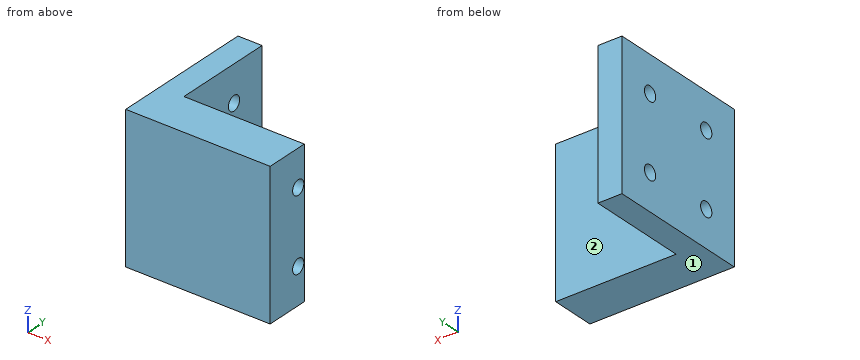
```python
from build123d import *

# Parameters (mm, degrees)
SKETCH1_W            = 60
SKETCH1_H            = 60
BOSS_EXTRUDE1_DEPTH  = 60
SKETCH2_R            = 3
CUT_EXTRUDE1_DEPTH   = 61
LPATTERN1_COUNT      = 2
LPATTERN1_PITCH      = 30
LPATTERN1_COUNT_DIR2 = 2
LPATTERN1_PITCH_DIR2 = 30
CUT_EXTRUDE3_REACH   = 62
SKETCH4_W            = 40
SKETCH4_H            = 41.75
CUT_EXTRUDE5_REACH   = 62
SKETCH6_W            = 10
SKETCH6_H            = 41.75


with BuildPart() as part:
    # Sketch1 → Boss-Extrude1 (new body)
    with BuildSketch(Plane(origin=(0, 0, 0), x_dir=(1, 0, 0), z_dir=(0, 1, 0))):
        Rectangle(SKETCH1_W, SKETCH1_H)
    extrude(amount=BOSS_EXTRUDE1_DEPTH)

    # Sketch2 → Cut-Extrude1 (cut, through all)
    with BuildSketch(Plane(origin=(30, 0, 0), x_dir=(0, 0, -1), z_dir=(1, 0, 0))):
        with Locations((-15, 45)):
            Circle(SKETCH2_R)
    cut_extrude1 = extrude(amount=-CUT_EXTRUDE1_DEPTH, mode=Mode.SUBTRACT)

    # LPattern1: Cut-Extrude1 2 × 2
    with Locations(*[(0, -j * LPATTERN1_PITCH_DIR2, -i * LPATTERN1_PITCH) for i in range(LPATTERN1_COUNT) for j in range(LPATTERN1_COUNT_DIR2) if (i, j) != (0, 0)]):
        add(cut_extrude1, mode=Mode.SUBTRACT)

    # Sketch4 → Cut-Extrude3 (cut, up to next)
    with BuildSketch(Plane(origin=(0, 0, -30), x_dir=(-1, 0, 0), z_dir=(0, 0, -1)), mode=Mode.PRIVATE) as cut_extrude3_sk1:
        with Locations((0, 39.125)):
            Rectangle(SKETCH4_W, SKETCH4_H)
    cut_extrude3_tool1 = extrude(cut_extrude3_sk1.sketch, amount=-CUT_EXTRUDE3_REACH, mode=Mode.PRIVATE) & part.part
    add(cut_extrude3_tool1.solids().sort_by_distance((0, 39.125, -30))[0], mode=Mode.SUBTRACT)

    # Sketch6 → Cut-Extrude5 (cut, up to next)
    with BuildSketch(Plane.XY.offset(30), mode=Mode.PRIVATE) as cut_extrude5_sk1:
        with Locations((25, 39.125)):
            Rectangle(SKETCH6_W, SKETCH6_H)
    cut_extrude5_tool1 = extrude(cut_extrude5_sk1.sketch, amount=-CUT_EXTRUDE5_REACH, mode=Mode.PRIVATE) & part.part
    add(cut_extrude5_tool1.solids().sort_by_distance((25, 39.125, 30))[0], mode=Mode.SUBTRACT)


solid = part.part
```
Here's how the part is built. I have some questions about the finished solid (model axes, mm). Face numbers are marked on the shaded views. A direction names the side the tool comes from. Coordinates: 2 decimals unless noted, no trailing zeros. Loops run counter-clockwise (first coordinate to the right, second up) from the corner with the lowest first, then second, coordinate; pieces in that order, holes last. Notation, with made-up numbers: (31, 17) - (45, 17) arc R21 ccw to (45, 31) - close; hole circle Ø6 at (-11.5, 7.25). An arc over 180 degrees is marked (long way). Return JSON: item names as keys, results as strings. Group by question number.
Item 1: If we section it at A-A on y = 15: Write out the boundary of the cut face in (x, z).
Item 2: Will these pins go through, and if not, where does the flat tip stop? P1, Ø8, axis at y = 45, z = -15, coming from the +X side; P2, Ø3, axis at x = -7.5, z = 20.5, coming from the +Y side.
Item 3: If we section it at B-B on z = 15: Write out the boundary of the cut face in (x, y), and give its area (3 significant figures).
Item 4: I need wall thicknesses on line 1 (Y direction, x = -26.75, z = -15); line 2 (X direction, y = 50, z = 3.5); line 3 (Y direction, x = 7, z = 15). Which ranges of each line are inside material? Lowest first, please. Write a range as from..to.
Item 5: On a 3-axis mill with a long thin cutter (end or side, diameter ignored), from which of +Z, -Z, +X, -X, +Y, -Y can I reach the whole of each face in a straight line? I mean the marked faces 1 and 2. Say none if no direction works.
Item 6: If we section it at D-D on y = 45: Write out the boundary of the cut face in (x, z).
Item 7: If we section it at C-C on x = 11: Write out the boundary of the cut face in (y, z), and give its area (3 significant figures).
Calculated:
{
 "1": {"outline": "(-30, -30) - (30, -30) - (30, -18) - (-30, -18) - close; (-30, -12) - (30, -12) - (30, 12) - (-30, 12) - close; (-30, 18) - (30, 18) - (30, 30) - (-30, 30) - close"},
 "2": {"P1": "stops at x = -20", "P2": "stops at y = 18.25"},
 "3": {"outline": "(-30, 0) - (30, 0) - (30, 12) - (-30, 12) - close; (-30, 18) - (30, 18) - (30, 18.25) - (-20, 18.25) - (-20, 42) - (-30, 42) - close; (-30, 48) - (-20, 48) - (-20, 60) - (-30, 60) - close", "area": "1,090 mm^2"},
 "4": {"line 1": "y = 0..12, 18..42, 48..60", "line 2": "x = -30..-20", "line 3": "y = 0..12, 18..18.25"},
 "5": {"face 1": "-Z, +X, -X, +Y, -Y", "face 2": "+Z, -Z, +X, +Y"},
 "6": {"outline": "(-30, -30) - (-20, -30) - (-20, -18) - (-30, -18) - close; (-30, -12) - (-20, -12) - (-20, 12) - (-30, 12) - close; (-30, 18) - (-20, 18) - (-20, 30) - (-30, 30) - close"},
 "7": {"outline": "(0, -30) - (18.25, -30) - (18.25, 30) - (0, 30) - close; hole circle Ø6 at (15, -15); hole circle Ø6 at (15, 15)", "area": "1,040 mm^2"}
}
